Autodesk Inventor part; units mm, degrees
ref_plane "YZ Plane" through (0, 0, 0) normal (1, 0, 0) x (0, 1, 0)
ref_plane "XZ Plane" through (0, 0, 0) normal (0, 1, 0) x (-1, 0, 0)
ref_plane "XY Plane" through (0, 0, 0) normal (0, 0, 1) x (1, 0, 0)
sketch "Sketch1" plane through (0, 0, 0) normal (0, 0, 1) x (1, 0, 0)
  line L0 (-12, -5) -> (12, -5)
  line L1 (12, -5) -> (12, 5)
  line L2 (12, 5) -> (-12, 5)
  line L3 (-12, 5) -> (-12, -5)
  line L4 (-12, -5) -> (12, 5) construction
  line L5 (12, -5) -> (-12, 5) construction
  line L6 (-12, 5) -> (-10, 5)
  line L7 (-12, 3) -> (-12, 5)
  line L8 (12, 5) -> (10, 5)
  line L9 (12, 3) -> (12, 5)
  circle A0 centre (-9.1253, 1.7977) radius 1.25
  circle A1 centre (9.1253, 1.7977) radius 1.25
  point P0 (0, 0)
  point P1 (-12, 0)
  point P2 (12, 0)
  point P3 (10.3753, 1.7977)
  point P4 (10.375, 1.7725)
  point P5 (9.4672, 3)
  point P6 (-9.4672, 3)
  point P7 (10.375, 1.7725)
  point P8 (-10.375, 1.7725)
  dimension "d0" = 24
  dimension "d1" = 10
  dimension "d14" = 2.5
  dimension "d15" = 2.5
  dimension "d55" = 8
  dimension "d58" = 8
  dimension "d60" = 1.625
  dimension "d61" = 1.625
  dimension "d62" = 18.2505
extrude "Extrusion4" add sketch "Sketch1" along normal blind 3
sketch "Sketch3" plane through (0, 0, 3) normal (0, 0, 1) x (1, 0, 0)
  line L0 (12, -5) -> (12, 5)
  line L1 (12, -5) -> (-12, -5)
  line L2 (-12, -5) -> (-12, -2)
  line L3 (-12, -2) -> (12, -2)
  line L4 (12, -2) -> (12, -5)
  point P0 (0, 0)
  point P1 (-12, -5)
  point P2 (12, 3)
  dimension "d24" = 3
extrude "Extrusion5" add sketch "Sketch3" along normal blind 27
sketch "Sketch4" plane through (-12, -2, 3) normal (0, 1, 0) x (1, 0, 0)
  circle A0 centre (22.625, -18.0021) radius 1
  circle A1 centre (1.375, -18.0021) radius 1
  circle A2 centre (22.625, -5.5021) radius 1
  circle A3 centre (1.375, -5.5021) radius 1
  line L0 (24, -0.0021) -> (0, -0.0021)
  line L1 (24, 0) -> (24, -27)
  line L2 (0, 3) -> (0, -27)
  point P0 (12, 3)
  dimension "d68" = 1.375
  dimension "d69" = 1.375
  dimension "d70" = 1.375
  dimension "d71" = 1.375
extrude "Extrusion7" cut sketch "Sketch4" against normal blind 3
sketch "Sketch5" plane through (0, 0, 0) normal (0, 0, -1) x (-1, 0, 0)
  circle A0 centre (-9.1253, 1.7977) radius 1.25
  circle A1 centre (9.1253, 1.7977) radius 1.25
  point P0 (0, 0)
sketch "Sketch6" plane through (-12, -5, 0) normal (-1, 0, 0) x (0, 0, 1)
  line L0 (0, 10) -> (0, 0)
  line L1 (0, 10) -> (3, 10)
  line L2 (0, 10) -> (3, 10)
  line L3 (3, 3) -> (3, 10)
  line L4 (3, 10) -> (3, 3)
  line L5 (30, 3) -> (30, 0)
  line L6 (3, 3) -> (30, 3)
  line L7 (30, 3) -> (30, 0)
  line L8 (30, 0) -> (0, 0)
  line L9 (0, 0) -> (0, 10)
  point P0 (0, 5)
extrude "Extrusion8" add sketch "Sketch6" along normal blind 2.75
sketch "Sketch7" plane through (12, -5, 0) normal (1, 0, 0) x (0, 0, -1)
  line L0 (0, 0) -> (0, 10)
  line L1 (0, 10) -> (-3, 10)
  line L2 (0, 10) -> (-3, 10)
  line L3 (-3, 3) -> (-3, 10)
  line L4 (-3, 10) -> (-3, 3)
  line L5 (-30, 0) -> (-30, 3)
  line L6 (-3, 3) -> (-30, 3)
  line L7 (-30, 3) -> (-30, 0)
  line L8 (0, 0) -> (-30, 0)
  line L9 (-30, 0) -> (0, 0)
  line L10 (0, 0) -> (0, 10)
  point P0 (0, 5)
extrude "Extrusion9" add sketch "Sketch7" along normal blind 2.75
properties part number "Kamera Holder"
Geometry: final body of the model. Coordinates: model frame, mm. A direction names the side the tool comes from. Give positions to 0.01 mm unless a question says otherwise; leave off trailing zeros. Order: outer loops, then holes, each group sorted by start corner. A loop starts at its lowest first (then second) coordinate and runs counter-clockwise, first axis right, second up. Notation, with made-up numbers: (-6, 57) -> (22, 57) arc R30 ccw to (22, 93) -> close; hole circle Ø4 at (27, 65). An arc over 180 degrees is marked (long way). Put each result on its own line as item: value.
Q1. Section C-C, the plane z = 26. Return loops of the section in (x, y).
Here are the results:
outline: (-14.75, -5) -> (14.75, -5) -> (14.75, -2) -> (-14.75, -2) -> close
Q2. Material intervals for L1, parallel to Y at x = 10, z = 6.75; L2, parallel to Z at x = -8.25, y = -1, sorted ascending.
Here are the results:
L1: y = -5 to -2
L2: z = 0 to 3
Q3. Pin query (flat end, axial travel): pin 1 (2.5 mm diameter, centred on x = 10.62, z = 8.5, fed in from -Y); pin 2 (3.5 mm diameter, centred on x = 5.5, y = 3, fed in from +Z); pin 3 (1.8 mm diameter, centred on x = -10.62, z = 21, fed in from -Y); pin 4 (2.5 mm diameter, centred on x = 10.62, z = 21, fed in from +Y). Return the tip coordinate at first contact, or that it passes through.
Here are the results:
pin 1: stops at y = -5
pin 2: stops at z = 3
pin 3: passes through
pin 4: stops at y = -2
Q4. Section A-A, the plane x = -6. Return loops of the section in (y, z).
Here are the results:
outline: (-5, 0) -> (5, 0) -> (5, 3) -> (-2, 3) -> (-2, 30) -> (-5, 30) -> close
Q5. Reachability of faces 1 (the face through (0, -2, 16)), 2 (the face through (-10.76, -3.48, 20.01)) from +Z, -Z, +X, -X, +Y, -Y: full face, straight path, thin tool, end or side. Return the list, or none.
Here are the results:
face 1: +Z, +X, -X, +Y
face 2: +Y, -Y
Q6. Section B-B, the plane y = -1.25. Return loops of the section in (x, z).
Here are the results:
outline: (-14.75, 0) -> (14.75, 0) -> (14.75, 3) -> (-14.75, 3) -> close
Q7. Draft query along X for faces 3 (the face through (9.888, -3.479, 7.826)), 4 (the face through (14.75, -2.2, 11.9)), 5 (the face through (10.49, -3.48, 20.01)), 6 (the face through (0, 5, 1)). Return one class per face: released by +X, released by -X, zero draft, split by the parting line, or undercut.
Here are the results:
face 3: undercut
face 4: released by +X
face 5: undercut
face 6: zero draft
